Geometry check sheet. Reference: the model listing, model coordinates, mm. Give positions to 0.01 mm unless a question says otherwise; leave off trailing zeros. Order: outer loops, then holes, each group sorted by start corner. A loop starts at its lowest first (then second) coordinate and runs counter-clockwise, first axis right, second up. Notation, with made-up numbers: (59.25, -29) - (116.25, -29) arc R22 ccw to (116.25, -8) - close; hole circle Ø11 at (1, -35.75). An arc over 180 degrees is marked (long way). Put each result on its own line as item: value. Start each with the question number.
Solid Edge part; units mm, degrees
sketch "Sketch1" plane through (0, 0, 0) normal (0, 0, 1) x (1, 0, 0)
  line L0 (0, 0) -> (0, 38.1)
  line L1 (0, 38.1) -> (123.825, 38.1)
  line L2 (123.825, 38.1) -> (123.825, 0)
  line L3 (123.825, 0) -> (0, 0)
  dimension "D1" = 123.825
extrude "Protrusion1" add sketch "Sketch1" along normal blind 6.35
hole "Hole_1" at (119.0625, 25.4, 6.35) direction (0, 0, -1) diameter 4.826 end up to next countersink diameter 9.525 countersink angle 82
hole "Hole1" at (4.7625, 25.4, 6.35) direction (0, 0, -1) diameter 4.826 end up to next countersink diameter 9.525 countersink angle 82
properties part number "CHAS-03"
Item 1: Cross-section at A-A (z = 5.25). Enter the section's corners in (x, y) (1 decimal).
Item 2: Release check for a two-part mould opening along Y. For faces 1 (the face through (123.825, 19, 3)), 2 (the face through (119.17, 27.81, 1.85)), 3 (the face through (61, 38.1, 3)), 4 (the face through (63, 0, 3)) record: +Y half, -Y half, draft (parallel to the pull), parting line (faces both ways), or undercut.
Item 3: Thickness scan on line 1 along X through (y, z) = (25.4, 2.6) (1 decimal); line 2 along X through (y, z) = (25.5, 4.25) (3 decimals). Record the ranges inside material, lowest first.
Item 4: Gauge pin test, flat ends, axial feed: pin 1 Ø5.5 at (x, y) = (4.76, 25.4) entering from +Z; pin 2 Ø6.5 at (x, y) = (119.06, 25.4) entering from +Z. Record the tip position at first contact, or that the pin passes through.
Recorded:
1. outline: (0, 0) - (123.8, 0) - (123.8, 38.1) - (0, 38.1) - close; hole circle Ø7.6 at (4.8, 25.4); hole circle Ø7.6 at (119.1, 25.4)
2. face 1: draft
2. face 2: undercut
2. face 3: +Y half
2. face 4: -Y half
3. line 1: x = 0 to 2.3, 7.2 to 116.6, 121.5 to 123.8
3. line 2: x = 0 to 1.827, 7.698 to 116.127, 121.998 to 123.825
4. pin 1: stops at z = 4.04
4. pin 2: stops at z = 4.61
